The model under review builds one solid part; all positions refer to its coordinate system, in mm. Give positions to 0.01 mm unless a question says otherwise; leave off trailing zeros. Order: outer loops, then holes, each group sorted by start corner. A loop starts at its lowest first (then second) coordinate and runs counter-clockwise, first axis right, second up.
```python
from build123d import *

# Parameters (mm, degrees)
F1_DEPTH = 45
F2_R     = 5
F3_R     = 5


with BuildPart() as f1:
    # F0 (on Front) → F1 (new body)
    with BuildSketch(Plane.XZ):
        Polygon((-199.459287, 55.321917), (-248.504069, -250), (-205.278272, -250), (-79.926361, 55.321917), align=None)
    extrude(amount=F1_DEPTH)

    # F2
    f2_edges = [f1.edges().sort_by_distance(p)[0] for p in [
        (-223.981678, 0, -97.339041),
        (-226.891171, 0, -250),
        (-142.602317, 0, -97.339041),
        (-139.692824, 0, 55.321917),
    ]]
    fillet(f2_edges, radius=F2_R)

    # F3
    f3_edges = [f1.edges().sort_by_distance(p)[0] for p in [
        (-223.981678, -45, -97.339041),
        (-226.891171, -45, -250),
        (-142.602317, -45, -97.339041),
        (-139.692824, -45, 55.321917),
    ]]
    fillet(f3_edges, radius=F3_R)


solid = f1.part
```
1. To check wall thickness, follow line 1 (X direction, y = -11.5, z = -181); line 2 (Z direction, x = -191, y = -12.5); line 3 (Z direction, x = -155, y = -21). State the ranges of each line that lie inside material, in increasing order.
2. Take a section at A-A (y = -28). Write out the cut boundary in (x, z), and give its area (3 significant figures).
3. Insertion check: pin 1 (10 mm diameter, centred on x = -199, y = -19.5, fed in from -Z); pin 2 (8 mm diameter, centred on y = -16, z = -95, fed in from +X); pin 3 (2 mm diameter, centred on x = -205, z = 8.5, fed in from +Y). Each pin has a flat end and moves straight along its axis. Give the tip position at first contact, or say it passes through.
Answer:
1. line 1: x = -237.42 to -176.95
1. line 2: z = -215.22 to 55.32
1. line 3: z = -127.54 to 55.32
2. outline: (-248.5, -250) - (-205.28, -250) - (-79.93, 55.32) - (-199.46, 55.32) - close
2. area: 24,800 mm2
3. pin 1: stops at z = -246.89
3. pin 2: stops at x = -140
3. pin 3: stops at y = -0.44
